from build123d import *

# Parameters (mm, degrees)
SKETCH_1_W                   = 26
SKETCH_1_H                   = 10
EXTRUDE_1_DEPTH              = 5
EXTRUDE_START                = 3.5
EXTRUDE_2_DEPTH              = 5
HOLE_WIZARD_M4_1_REACH       = 37.089
HOLE_WIZARD_M4_1_BORE_R      = 2.15
HOLE_WIZARD_M4_1_2_OUTLINE_R = 1.65
HOLE_WIZARD_M4_1_2_DEPTH     = 5
HOLE_WIZARD_M4_2_D           = 3.3


# Read off the part's stored shape, not the designer's step: M4 螺纹孔1
with BuildPart() as part:
    # 草图1 → 凸台-拉伸1 (new body)
    with BuildSketch(Plane(origin=(0, 0, 0), x_dir=(1, 0, 0), z_dir=(0, 1, 0))):
        Rectangle(SKETCH_1_W, SKETCH_1_H)
    extrude(amount=EXTRUDE_1_DEPTH)

    # 草图2 → 凸台-拉伸2 (add)
    with BuildSketch(Plane(origin=(0, 0, 0), x_dir=(0, 0, -1), z_dir=(1, 0, 0)).offset(EXTRUDE_START)):
        with BuildLine():
            Line((-5, 5), (5, 5))
            ThreePointArc((5, 5), (2.918749068, 17.246562174), (-3.091314031, 28.118040089))
            ThreePointArc((-3.091314031, 28.118040089), (-10.118040089, 28.908685969), (-10.908685969, 21.881959911))
            ThreePointArc((-10.908685969, 21.881959911), (-6.519834496, 13.943057927), (-5, 5))
        make_face()
    extrude_2 = extrude(amount=EXTRUDE_2_DEPTH)

    # 镜向1: 凸台-拉伸2 across plane
    add(extrude_2.mirror(Plane(origin=(0, 0, 0), x_dir=(0, 0, 1), z_dir=(1, 0, 0))))

    # Hole Wizard M4 _1 bore (on position points) → Hole Wizard M4 _1 (cut, up to next)
    with BuildSketch(Plane(origin=(8.5, 25, 7), x_dir=(0, 0, 1), z_dir=(1, 0, 0)), mode=Mode.PRIVATE) as hole_wizard_m4_1_sk1:
        Circle(HOLE_WIZARD_M4_1_BORE_R)
    hole_wizard_m4_1_tool1 = extrude(hole_wizard_m4_1_sk1.sketch, amount=-HOLE_WIZARD_M4_1_REACH, mode=Mode.PRIVATE) & part.part
    add(hole_wizard_m4_1_tool1.solids().sort_by_distance((8.5, 25, 7))[0], mode=Mode.SUBTRACT)

    # Hole Wizard M4 _1 2 outline → Hole Wizard M4 _1 2 (cut)
    with BuildSketch(Plane(origin=(0, 0, 0), x_dir=(1, 0, 0), z_dir=(0, 1, 0))):
        with Locations((7, 1)):
            Circle(HOLE_WIZARD_M4_1_2_OUTLINE_R)
    extrude(amount=HOLE_WIZARD_M4_1_2_DEPTH, mode=Mode.SUBTRACT)

    # Hole Wizard M4 _1 2 2 outline → Hole Wizard M4 _1 2 2 (revolve, cut)
    with BuildSketch(Plane(origin=(-7, 0, -1), x_dir=(1, 0, 0), z_dir=(0, 0, 1))):
        Polygon((1.650000121, 4.999999927), (0, 5.991420021), (0, 0), (1.650000121, 0), align=None)
    revolve(axis=Axis((-7, 0, -1), (0, 1, 0)), mode=Mode.SUBTRACT)

    # M4 螺纹孔2 (through all)
    with Locations(Plane.ZY.offset(8.5)):
        with Locations((7, 25)):
            Hole(HOLE_WIZARD_M4_2_D / 2)


solid = part.part
Model file for the job. Use its own axes, mm. A direction names the side the tool comes from. Give positions to 0.01 mm unless a question says otherwise; leave off trailing zeros. Loops run counter-clockwise (first coordinate to the right, second up) from the corner with the lowest first, then second, coordinate; pieces in that order, holes last.
Item 1: Slice it at A-A (x = 7). Write the cut outline in (y, z), plus the area to 3 significant figures.
Check values:
outline: (0, -5) - (5, -5) arc R37.07 ccw to (28.12, 3.09) arc R5 ccw to (21.88, 10.91) arc R27.07 cw to (5, 5) - (0, 5) - (0, 0.65) - (5, 0.65) - (5, -2.65) - (0, -2.65) - close; hole circle Ø4.3 at (25, 7)
area: 274 mm2
Item 2: Drop flat-ended pins along their axis: P1, Ø1.3, axis at x = -12, z = 0, coming from the +Y side; P2, Ø10, axis at y = 26, z = 6.5, coming from the +X side; P3, Ø3, axis at x = -7, z = -1, coming from the +Y side. Give the stop position or say it passes through.
Check values:
P1: stops at y = 5
P2: stops at x = 8.5
P3: stops at y = 24.43
Item 3: Drill centre lines: line 1 along X through (y, z) = (3.3, -1); line 2 along X through (y, z) = (6, 4.25); line 3 along Y through (x, z) = (-2.25, -0.75). Where is each one in solid material? Low to high.
Check values:
line 1: x = -13 to -8.65, -5.35 to 5.35, 8.65 to 13
line 2: x = -8.5 to -3.5, 3.5 to 8.5
line 3: y = 0 to 5
Item 4: Slice it at B-B (y = 16.5). Write the cut outline in (x, z).
Check values:
outline: (-8.5, -3.17) - (-3.5, -3.17) - (-3.5, 7.56) - (-8.5, 7.56) - close; (3.5, -3.17) - (8.5, -3.17) - (8.5, 7.56) - (3.5, 7.56) - close
Item 5: Which spindle directions (+Z, -Z, +X, -X, +Y, -Y) get a long thin tool onto all of the face, cutting with end or side? Do faces 1 (the face through (8.5, 18, 4)), 2 (the face through (-11, 5, 0)), 3 (the face through (0, 2, 5)), 4 (the face through (0, 5, 0)). Say none if no direction does.
Check values:
face 1: +Z, -Z, +X, +Y
face 2: +Z, -Z, -X, +Y
face 3: +Z, +X, -X, -Y
face 4: +Z, -Z, +Y
Item 6: Slice it at C-C (z = 9.5). Write the cut outline in (x, y).
Check values:
outline: (-8.5, 19.95) - (-3.5, 19.95) - (-3.5, 29.33) - (-8.5, 29.33) - close; (3.5, 19.95) - (8.5, 19.95) - (8.5, 29.33) - (3.5, 29.33) - close
Item 7: Slice it at D-D (y = 3.5). Write the cut outline in (x, z).
Check values:
outline: (-13, -5) - (13, -5) - (13, 5) - (-13, 5) - close; hole circle Ø3.3 at (-7, -1); hole circle Ø3.3 at (7, -1)
Item 8: Mould opens along X. For faces 5 (the face through (5.96, 14.06, 6.56)), 6 (the face through (-8.5, 18, 4)), 7 (the face through (-5.426, 2.535, -1.496)), 8 (the face through (5.35, 2.46, -1.07)) say: +X half, -X half, draft (parallel to the pull), parting line (faces both ways), or undercut.
Check values:
face 5: draft
face 6: -X half
face 7: undercut
face 8: undercut
